from build123d import *

# Parameters (mm, degrees)
FILLET1_R           = 10
SKETCH2_R           = 25
BOSS_EXTRUDE1_DEPTH = 80
CIRPATTERN1_COUNT   = 3


with BuildPart() as part:
    # Sketch1 → Revolve1 (revolve)
    with BuildSketch(Plane.XY):
        with BuildLine():
            Line((0, 214), (256, 214))
            Line((256, 214), (256, 284))
            Line((256, 284), (378, 284))
            Line((378, 284), (378, 146))
            ThreePointArc((378, 146), (392.644660941, 110.644660941), (428, 96))
            Line((428, 96), (466, 96))
            ThreePointArc((466, 96), (480.142135624, 90.142135624), (486, 76))
            Line((486, 76), (486, 0))
            ThreePointArc((486, 0), (400.474718303, -275.347053734), (174, -453.784089629))
            Line((174, -453.784089629), (0, -453.784089629))
            Line((0, -453.784089629), (0, 214))
        make_face()
    revolve(axis=Axis((0, -1000, 0), (0, 1, 0)))

    # Fillet1
    fillet1_edges = [part.edges().sort_by_distance(p)[0] for p in [
        (-256, 284, 0),
        (-378, 284, 0),
    ]]
    fillet(fillet1_edges, radius=FILLET1_R)

    # Sketch2 → Boss-Extrude1 (add)
    with BuildSketch(Plane.XZ.offset(453.784089629)):
        with Locations((-270, 0)):
            Circle(SKETCH2_R)
    boss_extrude1 = extrude(amount=-BOSS_EXTRUDE1_DEPTH)

    # CirPattern1: Boss-Extrude1 ×3 about axis
    cirpattern1_axis = Axis((0, 0, 0), (0, 1, 0))
    for i in range(1, CIRPATTERN1_COUNT):
        add(boss_extrude1.rotate(cirpattern1_axis, i * 360 / CIRPATTERN1_COUNT))


solid = part.part
Here's how the part is built. I have some questions about the finished solid (model axes, mm). A direction names the side the tool comes from. Coordinates: 2 decimals unless noted, no trailing zeros. Write each loop counter-clockwise with the first axis right and the second up, starting at its lowest first coordinate (ties: lowest second). Pieces come first, ordered by that corner, then holes.
Item 1: I want a section at A-A on x = 0. Write out the boundary of the cut face in (y, z).
Item 2: If I drill on line 1 (X direction, y = 258, z = 0); line 2 (X direction, y = -137, z = -20), over which ranges is the centre line in solid material (lowest first)?
Item 3: I want a section at C-C on y = 53. Write out the boundary of the cut face in (x, z), and give its area (3 significant figures).
Item 4: If we mould it in two halves opening along Z, with no side actions, what happens to faces 1 (the cylindrical face through (463.557, 37.468, -145.981)), 2 (the cylindrical face through (146.536, -427.985, -256.006)), 3 (the flat face through (-2, -453.784, -2))? For each: +Z half, -Z half, draft (parallel to the pull), parting line (faces both ways), or undercut.
Item 5: On a 3-axis mill with a long thin cutter (end or side, diameter ignored), from which of +Z, -Z, +X, -X, +Y, -Y can I reach the whole of each face in a straight line? I mean faces 4 (the flat face through (4, 214, -4)), 5 (the flat face through (135, -453.784, -234)). Say none if no direction works.
Item 6: Will these pins go through, and if not, where does the flat tip stop? pin 1 (3 mm diameter, centred on y = -257.5, z = 62.5, fed in from +X); pin 2 (3 mm diameter, centred on y = -183.5, z = -100, fed in from +X); pin 3 (12 mm diameter, centred on x = 271.5, z = 374.5, fed in from +Y).
Item 7: I want a section at B-B on z = 0. Write out the boundary of the cut face in (x, y).
Item 8: I want a section at D-D on y = 171.5. Write out the boundary of the cut face in (x, z), and give its area (3 significant figures).
Findings below:
1. outline: (-453.78, -174) arc R486 ccw to (0, -486) - (76, -486) arc R20 ccw to (96, -466) - (96, -428) arc R50 cw to (146, -378) - (274, -378) arc R10 ccw to (284, -368) - (284, -266) arc R10 ccw to (274, -256) - (214, -256) - (214, 256) - (274, 256) arc R10 ccw to (284, 266) - (284, 368) arc R10 ccw to (274, 378) - (146, 378) arc R50 cw to (96, 428) - (96, 466) arc R20 ccw to (76, 486) - (0, 486) arc R486 ccw to (-453.78, 174) - close
2. line 1: x = -378 to -256, 256 to 378
2. line 2: x = -465.86 to 465.86
3. outline: circle Ø972 at (0, 0)
3. area: 742,000 mm2
4. face 1: parting line
4. face 2: undercut
4. face 3: draft
5. face 4: +Y
5. face 5: +Z, -Z, +X, -X, -Y
6. pin 1: stops at x = 408.38
6. pin 2: stops at x = 439.49
6. pin 3: stops at y = 96
7. outline: (-486, 0) arc R486 ccw to (-295, -386.23) - (-295, -453.78) - (-245, -453.78) - (-245, -419.73) arc R486 ccw to (-174, -453.78) - (174, -453.78) arc R486 ccw to (486, 0) - (486, 76) arc R20 ccw to (466, 96) - (428, 96) arc R50 cw to (378, 146) - (378, 274) arc R10 ccw to (368, 284) - (266, 284) arc R10 ccw to (256, 274) - (256, 214) - (-256, 214) - (-256, 274) arc R10 ccw to (-266, 284) - (-368, 284) arc R10 ccw to (-378, 274) - (-378, 146) arc R50 cw to (-428, 96) - (-466, 96) arc R20 ccw to (-486, 76) - close
8. outline: circle Ø756 at (0, 0)
8. area: 449,000 mm2
